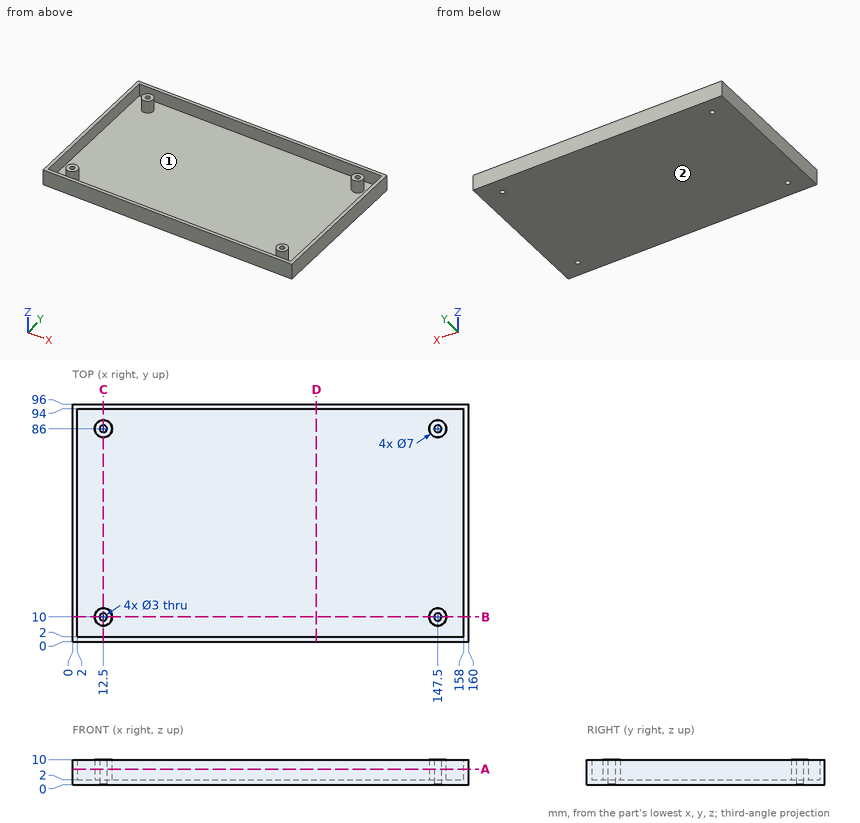
Check sheet for the drawn part. Datum: minimum x, y, z corner. Units: mm. Round coordinates to 2 decimals unless told otherwise and drop trailing zeros. Write each loop counter-clockwise with the first axis right and the second up, starting at its lowest first coordinate (ties: lowest second). Pieces come first, ordered by that corner, then holes. Notation, with made-up numbers: (69, 84) -> (119, 84) arc R25 cw to (119, 107) -> close; hole circle Ø11 at (58.25, -33.75). An arc over 180 degrees is marked (long way). Put each result on its own line as item: value.
(1) Sectioned sample at A-A (z = 6.25). Count the separate pieces of the cut face and the enclosed holes in it, plus the area to 3 significant figures.
Values found:
separate pieces: 5
enclosed holes: 5
area: 1,130 mm^2
(2) Material ranges on line 1 (Y direction, x = 12.5, z = 4); line 2 (X direction, y = 86, z = 2.75); line 3 (Y direction, x = 34, z = 4), recorded low to high.
Values found:
line 1: y = 0 to 2, 6.5 to 8.5, 11.5 to 13.5, 82.5 to 84.5, 87.5 to 89.5, 94 to 96
line 2: x = 0 to 2, 9 to 11, 14 to 16, 144 to 146, 149 to 151, 158 to 160
line 3: y = 0 to 2, 94 to 96
(3) Go/stop test with flat-tipped pins: pin 1 Ø6 at (x, y) = (122, 44) entering from +Z; pin 2 Ø1.8 at (x, y) = (12.5, 10) entering from -Z. Record where each tip stops, or that it passes through.
Values found:
pin 1: stops at z = 2
pin 2: passes through
(4) Sectioned sample at C-C (x = 12.5). Enter the section's corners in (y, z), plus the area to 3 significant figures.
Values found:
outline: (0, 0) -> (8.5, 0) -> (8.5, 10) -> (6.5, 10) -> (6.5, 2) -> (2, 2) -> (2, 10) -> (0, 10) -> close; (11.5, 0) -> (84.5, 0) -> (84.5, 10) -> (82.5, 10) -> (82.5, 2) -> (13.5, 2) -> (13.5, 10) -> (11.5, 10) -> close; (87.5, 0) -> (96, 0) -> (96, 10) -> (94, 10) -> (94, 2) -> (89.5, 2) -> (89.5, 10) -> (87.5, 10) -> close
area: 276 mm^2
(5) Sectioned sample at D-D (x = 98.5). Enter the section's corners in (y, z).
Values found:
outline: (0, 0) -> (96, 0) -> (96, 10) -> (94, 10) -> (94, 2) -> (2, 2) -> (2, 10) -> (0, 10) -> close
(6) Sectioned sample at B-B (y = 10). Enter the section's corners in (x, z), plus the area to 3 significant figures.
Values found:
outline: (0, 0) -> (11, 0) -> (11, 10) -> (9, 10) -> (9, 2) -> (2, 2) -> (2, 10) -> (0, 10) -> close; (14, 0) -> (146, 0) -> (146, 10) -> (144, 10) -> (144, 2) -> (16, 2) -> (16, 10) -> (14, 10) -> close; (149, 0) -> (160, 0) -> (160, 10) -> (158, 10) -> (158, 2) -> (151, 2) -> (151, 10) -> (149, 10) -> close
area: 404 mm^2
(7) Mould release check, pull along Y, two halves, no side actions. Record for the marked faces 1 and 2: released by +Y, released by -Y, zero draft, split by the parting line, or undercut.
Values found:
face 1: undercut
face 2: zero draft
